Build history of the part. All positions in model axes, mm. A direction names the side the tool comes from. Give positions to 0.01 mm unless a question says otherwise; leave off trailing zeros. Order: outer loops, then holes, each group sorted by start corner. A loop starts at its lowest first (then second) coordinate and runs counter-clockwise, first axis right, second up. Notation, with made-up numbers: M 72,34 L 112,34 A35 cw 112,69 Z; hole C -40,6 d10. An arc over 180 degrees is marked long. One line per item, written item: value. Start each with the question number.
from build123d import *

# Parameters (mm, degrees)
SKETCH_1_W          = 26
SKETCH_1_H          = 19
EXTRUDE_1_DEPTH     = 10
SKETCH_2_W          = 15.2
SKETCH_2_H          = 19
CUT_EXTRUDE_1_DEPTH = 4
CUT_EXTRUDE_2_DEPTH = 4
CHAMFER_1_SIZE      = 1
FILLET_1_R          = 1
SKETCH_4_R          = 1.1
CUT_EXTRUDE_3_DEPTH = 18.182840277
CUT_EXTRUDE_4_DEPTH = 3


with BuildPart() as part:
    # Эскиз1 → Бобышка-Вытянуть1 (new body)
    with BuildSketch(Plane(origin=(0, 0, 0), x_dir=(0, 0, -1), z_dir=(1, 0, 0))):
        Rectangle(SKETCH_1_W, SKETCH_1_H)
        with BuildLine():
            Line((-8.9, 6.5), (-8.9, -6.5))
            ThreePointArc((-8.9, -6.5), (-10, -7.6), (-11.1, -6.5))
            Line((-11.1, -6.5), (-11.1, 6.5))
            ThreePointArc((-11.1, 6.5), (-10, 7.6), (-8.9, 6.5))
        make_face(mode=Mode.SUBTRACT)
        with BuildLine():
            Line((8.9, 6.5), (8.9, -6.5))
            ThreePointArc((8.9, -6.5), (10, -7.6), (11.1, -6.5))
            Line((11.1, -6.5), (11.1, 6.5))
            ThreePointArc((11.1, 6.5), (10, 7.6), (8.9, 6.5))
        make_face(mode=Mode.SUBTRACT)
    extrude(amount=EXTRUDE_1_DEPTH)

    # Эскиз2 → Вырез-Вытянуть1 (cut)
    with BuildSketch(Plane(origin=(10, 0, 0), x_dir=(0, 0, -1), z_dir=(1, 0, 0))):
        Rectangle(SKETCH_2_W, SKETCH_2_H)
    extrude(amount=-CUT_EXTRUDE_1_DEPTH, mode=Mode.SUBTRACT)

    # Эскиз3 → Вырез-Вытянуть2 (cut)
    with BuildSketch(Plane(origin=(10, 0, 0), x_dir=(0, 0, -1), z_dir=(1, 0, 0))):
        with BuildLine():
            Line((-11.8, -6.5), (-11.8, 6.5))
            ThreePointArc((-11.8, 6.5), (-10, 8.3), (-8.2, 6.5))
            Line((-8.2, 6.5), (-8.2, -6.5))
            ThreePointArc((-8.2, -6.5), (-10, -8.3), (-11.8, -6.5))
        make_face()
        with BuildLine():
            Line((11.8, -6.5), (11.8, 6.5))
            ThreePointArc((11.8, 6.5), (10, 8.3), (8.2, 6.5))
            Line((8.2, 6.5), (8.2, -6.5))
            ThreePointArc((8.2, -6.5), (10, -8.3), (11.8, -6.5))
        make_face()
    extrude(amount=-CUT_EXTRUDE_2_DEPTH, mode=Mode.SUBTRACT)

    # Фаска1
    chamfer_1_edges = [part.edges().sort_by_distance(p)[0] for p in [
        (5, -9.5, -13),
        (5, -9.5, 13),
        (5, 9.5, 13),
        (5, 9.5, -13),
    ]]
    chamfer(chamfer_1_edges, length=CHAMFER_1_SIZE)

    # Скругление1
    fillet_1_edges = [part.edges().sort_by_distance(p)[0] for p in [
        (10, 9.5, -9.8),
        (10, 0, -13),
        (10, -9, -12.5),
        (10, 9, -12.5),
        (10, -9.5, 9.8),
        (10, 0, 13),
        (10, 9, 12.5),
        (10, -9, 12.5),
        (10, -9.5, -9.8),
        (10, 9.5, 9.8),
    ]]
    fillet(fillet_1_edges, radius=FILLET_1_R)

    # Эскиз4 → Вырез-Вытянуть3 (cut, through all)
    with BuildSketch(Plane(origin=(6, 0, 0), x_dir=(0, 0, -1), z_dir=(1, 0, 0))):
        with Locations((0, 5)):
            Circle(SKETCH_4_R)
        with Locations(Location((0, -5, 0), (0, 0, 180))):
            Circle(SKETCH_4_R)
    extrude(amount=-CUT_EXTRUDE_3_DEPTH, mode=Mode.SUBTRACT)

    # Эскиз5 → Вырез-Вытянуть4 (cut)
    with BuildSketch(Plane.ZY):
        Polygon((1.125833025, 3.05), (2.25166605, 5), (1.125833025, 6.95), (-1.125833025, 6.95), (-2.25166605, 5), (-1.125833025, 3.05), align=None)
        Polygon((1.125833025, -6.95), (2.25166605, -5), (1.125833025, -3.05), (-1.125833025, -3.05), (-2.25166605, -5), (-1.125833025, -6.95), align=None)
    extrude(amount=-CUT_EXTRUDE_4_DEPTH, mode=Mode.SUBTRACT)


solid = part.part
1) Pull direction Z, two halves, no side cores. Call faces 4 (the cylindrical face through (9.699, 9.215, -9.831)), 5 (the cylindrical face through (8, -8.3, 10)), 6 (the flat face through (4, 0, 13)): pulls with the +Z half, pulls with the -Z half, needs draft (parallel to the pull), parting line crosses it, or undercut.
2) Slice it at D-D (x = 5). List the corners of the cut face in (y, z).
3) Drill centre lines: line 1 (Z direction, x = 5.05, y = -5); line 2 (Z direction, x = 6.25, y = 6.25); line 3 (Y direction, x = 3.9, z = 0). Where is each one in solid material? Low to high.
4) Slice it at A-A (x = 1.25). List the corners of the cut face in (y, z).
5) Tool access for faces 1 (the flat face through (8, 0, 11.8)), 2 (the flat face through (1, 3.05, 0)), 3 (the cylindrical face through (3, 7.6, 10)): list every direction of +Z, -Z, +X, -X, +Y, -Y with a clear straight run to the whole face (end or side of a thin tool).
6) Slice it at B-B (z = -10). List the corners of the cut face in (x, y).
7) Slice it at C-C (y = -1). List the corners of the cut face in (x, z), plus the area to 3 significant figures.
8) Drop flat-ended pins along their axis: P1, Ø1.8, axis at y = -1, z = -10.5, coming from the +X side; P2, Ø4, axis at y = -1, z = 10.5, coming from the +X side; P3, Ø3, axis at y = -5, z = 0, coming from the -X side. Give the stop position or say it passes through.
Results list:
1. face 4: needs draft
1. face 5: undercut
1. face 6: pulls with the +Z half
2. outline: M -9.5,-12 L -8.5,-13 L 8.5,-13 L 9.5,-12 L 9.5,12 L 8.5,13 L -8.5,13 L -9.5,12 Z; hole M -6.5,-11.1 L 6.5,-11.1 A1.1 ccw 6.5,-8.9 L -6.5,-8.9 A1.1 ccw Z; hole M -6.5,8.9 L 6.5,8.9 A1.1 ccw 6.5,11.1 L -6.5,11.1 A1.1 ccw Z; hole C -5,0 d2.2; hole C 5,0 d2.2
3. line 1: z = -13 to -11.1, -8.9 to -1.1, 1.1 to 8.9, 11.1 to 13
3. line 2: z = -13 to -11.8, -8.2 to -7.6, 7.6 to 8.2, 11.8 to 13
3. line 3: y = -9.5 to -6.1, -3.9 to 3.9, 6.1 to 9.5
4. outline: M -9.5,-12 L -8.5,-13 L 8.5,-13 L 9.5,-12 L 9.5,12 L 8.5,13 L -8.5,13 L -9.5,12 Z; hole M -6.95,-1.13 L -5,-2.25 L -3.05,-1.13 L -3.05,1.13 L -5,2.25 L -6.95,1.13 Z; hole M -6.5,-11.1 L 6.5,-11.1 A1.1 ccw 6.5,-8.9 L -6.5,-8.9 A1.1 ccw Z; hole M -6.5,8.9 L 6.5,8.9 A1.1 ccw 6.5,11.1 L -6.5,11.1 A1.1 ccw Z; hole M 3.05,-1.13 L 5,-2.25 L 6.95,-1.13 L 6.95,1.13 L 5,2.25 L 3.05,1.13 Z
5. face 1: +X
5. face 2: -X
5. face 3: +X, -X
6. outline: M 0,-9.5 L 9,-9.5 A1 ccw 10,-8.5 L 10,-8.3 L 6,-8.3 L 6,-7.6 L 0,-7.6 Z; M 0,7.6 L 6,7.6 L 6,8.3 L 10,8.3 L 10,8.5 A1 ccw 9,9.5 L 0,9.5 Z
7. outline: M 0,-13 L 9,-13 A1 ccw 10,-12 L 10,-11.8 L 6,-11.8 L 6,-11.1 L 0,-11.1 Z; M 0,-8.9 L 6,-8.9 L 6,-8.2 L 10,-8.2 L 10,-7.6 L 6,-7.6 L 6,7.6 L 10,7.6 L 10,8.2 L 6,8.2 L 6,8.9 L 0,8.9 Z; M 0,11.1 L 6,11.1 L 6,11.8 L 10,11.8 L 10,12 A1 ccw 9,13 L 0,13 Z
7. area: 144 mm²
8. P1: stops at x = 6
8. P2: stops at x = 10
8. P3: stops at x = 3
